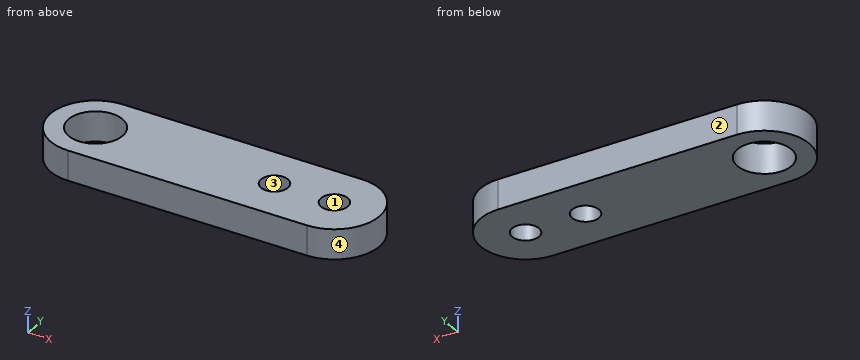
Autodesk Inventor part; units mm, degrees
ref_plane "YZ Plane" through (0, 0, 0) normal (1, 0, 0) x (0, 1, 0)
ref_plane "XZ Plane" through (0, 0, 0) normal (0, 1, 0) x (-1, 0, 0)
ref_plane "XY Plane" through (0, 0, 0) normal (0, 0, 1) x (1, 0, 0)
ref_plane "Work Plane1" through (88.049, 6.8107, 7.4208) normal (0, 0, 1) x (0, -1, 0)
sketch "Sketch1" plane through (88.049, 6.8107, 7.4208) normal (0, 0, 1) x (0, -1, 0)
  circle A0 centre (8.5, 0) radius 2.55 construction
  line L0 (38.25, 32.75) -> (-21.25, 32.75)
  circle A1 centre (8.5, -19.85) radius 4 construction
  line L1 (8.5, -19.85) -> (8.5, 20) construction
  line L2 (16, -19.85) -> (16, 20)
  line L3 (1, 20) -> (1, -19.85)
  arc A2 (1, -19.85) -> (16, -19.85) centre (8.5, -19.85) ccw
  arc A3 (16, 20) -> (1, 20) centre (8.5, 20) ccw
  point P0 (6.8107, -88.049)
  point P1 (8.5, 0.075)
  dimension "d0" = 15
  dimension "d20" = 20
extrude "Extrusion1" add sketch "Sketch1" along normal blind 5
sketch "Sketch2" plane through (88.049, 6.8107, 12.4208) normal (0, 0, 1) x (1, 0, 0)
  circle A0 centre (-19.85, -8.5) radius 4 construction
  circle A1 centre (0, -8.5) radius 2.55 construction
  line L0 (0, -8.5) -> (22.0742, -8.5) construction
  point P0 (-88.049, -6.8107)
  point P1 (10, -8.5)
  point P2 (20, -8.5)
  dimension "d4" = 10
  dimension "d5" = 10
hole "Hole1" at (98.049, -1.6893, 12.4208) at (108.049, -1.6893, 12.4208) direction (0, 0, -1) diameter 4.5 depth 6
sketch "Sketch3" plane through (88.049, 6.8107, 12.4208) normal (0, 0, 1) x (1, 0, 0)
  point P0 (-88.049, -6.8107)
  point P1 (-19.85, -8.5)
hole "Hole2" at (68.199, -1.6893, 12.4208) direction (0, 0, -1) diameter 9 depth 6
properties part number "GantryAxisHolder"
Verification items for the finished model (mm, model axes). Face numbers are marked on the shaded views. Round coordinates to 2 decimals unless told otherwise and drop trailing zeros. Order: outer loops, then holes, each group sorted by start corner. A loop starts at its lowest first (then second) coordinate and runs counter-clockwise, first axis right, second up. Notation, with made-up numbers: (55.25, 55) -> (88.25, 55) arc R25 cw to (88.25, 75) -> close; hole circle Ø5 at (-23.5, -39). An arc over 180 degrees is marked (long way). Put each result on its own line as item: value.
1) Section check D-D (x = 97.5). Record the cut outline in (y, z), then the cut area to 3 significant figures.
Final values:
outline: (-9.19, 7.42) -> (-3.87, 7.42) -> (-3.87, 12.42) -> (-9.19, 12.42) -> close; (0.49, 7.42) -> (5.81, 7.42) -> (5.81, 12.42) -> (0.49, 12.42) -> close
area: 53.2 mm^2
2) Material ranges on line 1 (X direction, y = -1.5, z = 9); line 2 (X direction, y = -3.5, z = 9.3); line 3 (X direction, y = 1.5, z = 10.25), recorded low to high.
Final values:
line 1: x = 60.7 to 63.7, 72.7 to 95.81, 100.29 to 105.81, 110.29 to 115.55
line 2: x = 60.92 to 64.08, 72.32 to 96.71, 99.38 to 106.71, 109.38 to 115.33
line 3: x = 61.41 to 65.02, 71.37 to 114.84
3) Section check A-A (x = 71). Record the cut outline in (y, z), then the cut area to 3 significant figures.
Final values:
outline: (-9.19, 7.42) -> (-5.21, 7.42) -> (-5.21, 12.42) -> (-9.19, 12.42) -> close; (1.83, 7.42) -> (5.81, 7.42) -> (5.81, 12.42) -> (1.83, 12.42) -> close
area: 39.8 mm^2
4) Section check B-B (y = -2.25). Record the cut outline in (x, z).
Final values:
outline: (60.72, 7.42) -> (63.73, 7.42) -> (63.73, 12.42) -> (60.72, 12.42) -> close; (72.66, 7.42) -> (95.87, 7.42) -> (95.87, 12.42) -> (72.66, 12.42) -> close; (100.23, 7.42) -> (105.87, 7.42) -> (105.87, 12.42) -> (100.23, 12.42) -> close; (110.23, 7.42) -> (115.53, 7.42) -> (115.53, 12.42) -> (110.23, 12.42) -> close
5) Section check C-C (z = 11). Record the cut outline in (x, y), then the cut area to 3 significant figures.
Final values:
outline: (68.2, -9.19) -> (108.05, -9.19) arc R7.5 ccw to (108.05, 5.81) -> (68.2, 5.81) arc R7.5 ccw to start; hole circle Ø9 at (68.2, -1.69); hole circle Ø4.5 at (98.05, -1.69); hole circle Ø4.5 at (108.05, -1.69)
area: 679 mm^2
6) Mould release check, pull along Y, two halves, no side actions. Record for the marked faces 1, 2, 3 and 4: +Y half, -Y half, draft (parallel to the pull), parting line (faces both ways), or undercut.
Final values:
face 1: undercut
face 2: +Y half
face 3: undercut
face 4: parting line
